Design review of the part shown in the three views and the two pictorial views. Dimensions are in mm from the part's minimum x, y and z. A direction names the side the tool comes from. Give positions to 0.01 mm unless a question says otherwise; leave off trailing zeros. Order: outer loops, then holes, each group sorted by start corner. A loop starts at its lowest first (then second) coordinate and runs counter-clockwise, first axis right, second up.
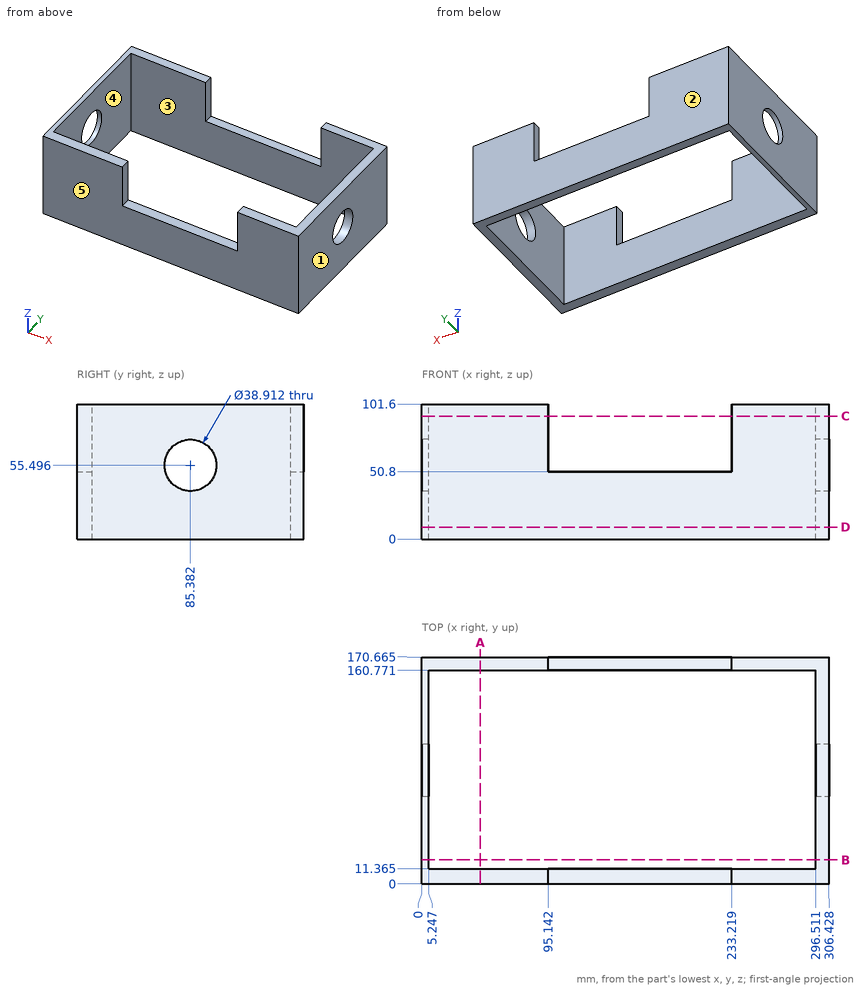
1) Tool access review of the marked faces 4 and 5: name each direction out of +Z, -Z, +X, -X, +Y, -Y from which nothing blocks a thin tool from reaching the whole face with its end or side.
Answer sheet:
face 4: +Z, -Z
face 5: +Z, -Z, +X, -X, -Y
2) We need section A-A on x = 44. Give the boundary of the cut face in (y, z) (1 decimal), then the cut area to 3 significant figures.
Answer sheet:
outline: (0, 0) - (11.4, 0) - (11.4, 101.6) - (0, 101.6) - close; (160.8, 0) - (170.7, 0) - (170.7, 101.6) - (160.8, 101.6) - close
area: 2,160 mm2
3) Draft analysis for pull direction X (two halves, no side actions). For the marked faces 1, 2 and 3, state which applies: +X half, -X half, draft (parallel to the pull), parting line (faces both ways), or undercut.
Answer sheet:
face 1: +X half
face 2: draft
face 3: undercut
4) Clearance check with flat-ended pins moving along their axes: pin 1 (5.5 mm diameter, centred on x = 153, y = 5.5, fed in from +Z); pin 2 (12 mm diameter, centred on x = 135.5, z = 61.5, fed in from -Y). State where each tip first meets the part, or that it passes through.
Answer sheet:
pin 1: stops at z = 50.8
pin 2: passes through
5) We need section C-C on z = 92.5. Give the boundary of the cut face in (x, y) (1 decimal).
Answer sheet:
outline: (0, 0) - (95.1, 0) - (95.1, 11.4) - (5.2, 11.4) - (5.2, 160.8) - (95.1, 160.8) - (95.1, 170.7) - (0, 170.7) - close; (233.2, 0) - (306.4, 0) - (306.4, 170.7) - (233.2, 170.7) - (233.2, 160.8) - (296.5, 160.8) - (296.5, 11.4) - (233.2, 11.4) - close
6) We need section D-D on z = 9. Give the boundary of the cut face in (x, y) (1 decimal), then the cut area to 3 significant figures.
Answer sheet:
outline: (0, 0) - (306.4, 0) - (306.4, 170.7) - (0, 170.7) - close; hole (5.2, 11.4) - (296.5, 11.4) - (296.5, 160.8) - (5.2, 160.8) - close
area: 8,780 mm2
7) We need section B-B on y = 18. Give the boundary of the cut face in (x, z), then the cut area to 3 significant figures.
Answer sheet:
outline: (0, 0) - (5.25, 0) - (5.25, 101.6) - (0, 101.6) - close; (296.51, 0) - (306.43, 0) - (306.43, 101.6) - (296.51, 101.6) - close
area: 1,540 mm2
8) To check wall thickness, follow line 1 (X direction, y = 28, z = 47); line 2 (Y direction, x = 275, z = 76) (1 decimal); line 3 (Z direction, x = 177, y = 164.5). State the ranges of each line that lie inside material, in increasing order.
Answer sheet:
line 1: x = 0 to 5.25, 296.51 to 306.43
line 2: y = 0 to 11.4, 160.8 to 170.7
line 3: z = 0 to 50.8
